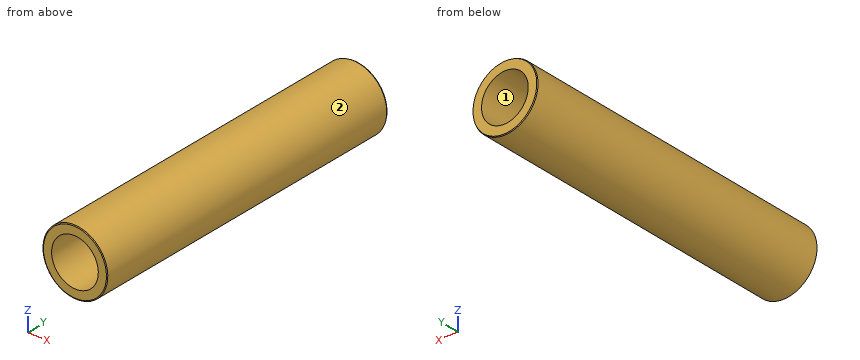
from build123d import *
from OCP.BRepFilletAPI import BRepFilletAPI_MakeChamfer

# Parameters (mm, degrees)
SKETCH1_R           = 60
BOSS_EXTRUDE1_DEPTH = 600
SKETCH2_R           = 43.239378985
CUT_EXTRUDE1_DEPTH  = 606.970296302
CHAMFER1_SIZE       = 1.674878
CHAMFER1_SIZE2      = 0.966991


with BuildPart() as part:
    # Sketch1 → Boss-Extrude1 (new body)
    with BuildSketch(Plane(origin=(0, 0, 0), x_dir=(1, 0, 0), z_dir=(0, 1, 0))):
        with Locations(Location((0, 0, 0), (0, 0, 270))):
            Circle(SKETCH1_R)
    extrude(amount=BOSS_EXTRUDE1_DEPTH)

    # Sketch2 → Cut-Extrude1 (cut, through all)
    with BuildSketch(Plane(origin=(0, 0, 0), x_dir=(1, 0, 0), z_dir=(0, 1, 0))):
        with Locations(Location((0, 0, 0), (0, 0, 270))):
            Circle(SKETCH2_R)
    extrude(amount=CUT_EXTRUDE1_DEPTH, mode=Mode.SUBTRACT)

    # Chamfer1: one chamfer whose edges measure the first distance from different faces: ONE call of the kernel's chamfer builder (chamfer() names one face for all edges)
    chamfer1_edges_1 = [part.edges().sort_by_distance(p)[0] for p in [
        (0, 0, -60),
    ]]
    chamfer1_side_1 = [part.faces().sort_by_distance(p)[0] for p in [
        (0, 0, -58.302943725),
    ]]
    chamfer1_edges_2 = [part.edges().sort_by_distance(p)[0] for p in [
        (0, 600, -60),
    ]]
    chamfer1_side_2 = [part.faces().sort_by_distance(p)[0] for p in [
        (0, 300, -60),
    ]]
    chamfer1 = BRepFilletAPI_MakeChamfer(part.part.solid().wrapped)
    for e in chamfer1_edges_1:
        chamfer1.Add(CHAMFER1_SIZE, CHAMFER1_SIZE2, e.wrapped, chamfer1_side_1[0].wrapped)  # the first distance lies on this face
    for e in chamfer1_edges_2:
        chamfer1.Add(CHAMFER1_SIZE, CHAMFER1_SIZE2, e.wrapped, chamfer1_side_2[0].wrapped)  # the first distance lies on this face
    add(Compound.cast(chamfer1.Shape()), mode=Mode.REPLACE)


solid = part.part
For this review, take the finished solid that the model builds, in its own axes (mm). Face numbers are marked on the shaded views. Round coordinates to 2 decimals unless told otherwise and drop trailing zeros. Order: outer loops, then holes, each group sorted by start corner. A loop starts at its lowest first (then second) coordinate and runs counter-clockwise, first axis right, second up. Notation, with made-up numbers: (49.25, -4) -> (87.25, -4) arc R18 ccw to (87.25, 15) -> close; hole circle Ø6 at (53.25, -39.5). An arc over 180 degrees is marked (long way). Put each result on its own line as item: value.
Q1. Mouldability with a two-part tool opening along Z and no side actions: class the marked faces 1 and 2 as pulls with the +Z half, pulls with the -Z half, needs draft (parallel to the pull), parting line crosses it, or undercut.
Check result:
face 1: undercut
face 2: parting line crosses it
Q2. Add section A-A on x = 0. Write out the cut boundary in (y, z), plus the area to 3 significant figures.
Check result:
outline: (0, -58.33) -> (0.97, -60) -> (598.33, -60) -> (600, -59.03) -> (600, -43.24) -> (0, -43.24) -> close; (0, 43.24) -> (600, 43.24) -> (600, 59.03) -> (598.33, 60) -> (0.97, 60) -> (0, 58.33) -> close
area: 20,100 mm2
Q3. For probe 1 along X at (y, z) = (136, 0); probe 2 along Z at (x, y) = (18.5, 63); probe 3 along Z at (x, y) = (-11, 414.5), list the stretches that pass through material, from the lowest coordinate up. Write a range as [from, to].
Check result:
probe 1: [-60, -43.24], [43.24, 60]
probe 2: [-57.08, -39.08], [39.08, 57.08]
probe 3: [-58.98, -41.82], [41.82, 58.98]
Q4. Insertion check: pin 1 Ø4 at (x, y) = (14, 524) entering from +Z; pin 2 Ø4 at (y, z) = (434, -3.5) entering from +X; pin 3 Ø4 at (y, z) = (293, -37) entering from -X. Each pin has a flat end and moves straight along its axis. Give the tip position at first contact, or say it passes through.
Check result:
pin 1: z = 58.79
pin 2: x = 59.98
pin 3: x = -48.73
Q5. Add section C-C on y = 406.5. Write out the cut boundary in (x, z).
Check result:
outline: circle Ø120 at (0, 0); hole circle Ø86.48 at (0, 0)
Q6. Add section B-B on z = 0. Write out the cut boundary in (x, y).
Check result:
outline: (-60, 0.97) -> (-58.33, 0) -> (-43.24, 0) -> (-43.24, 600) -> (-59.03, 600) -> (-60, 598.33) -> close; (43.24, 0) -> (58.33, 0) -> (60, 0.97) -> (60, 598.33) -> (59.03, 600) -> (43.24, 600) -> close
